Input: part model. Units: mm. Frame: model coordinates. Face numbers are marked on the shaded views. Coordinates: 2 decimals unless noted, no trailing zeros. Loops run counter-clockwise (first coordinate to the right, second up) from the corner with the lowest first, then second, coordinate; pieces in that order, holes last. Notation, with made-up numbers: M -5.75,16.25 L 26.25,16.25 A29 cw 26.25,42.25 Z; hole C -19,-20 d11. An arc over 180 degrees is marked long. Use a Markdown table: item, result. Add a question column.
1. Pin query (flat end, axial travel): pin 1 (7.5 mm diameter, centred on x = 7.5, z = 1.5, fed in from +Y). Return the tip coordinate at first contact, or that it passes through.
2. Section B-B on z = 0. Output: boundary loops of the cut face in (x, y), then the cut area to 3 significant figures.
3. Section A-A on y = 64.5. Output: boundary loops of the cut face in (x, z).
4. Section D-D on y = 47. Output: boundary loops of the cut face in (x, z).
5. Draft query along X for the marked faces 1, 2, 3 and 4. Return one class per face: +X half, -X half, draft (parallel to the pull), parting line (faces both ways), or undercut.
6. Section C-C on x = 17. Output: boundary loops of the cut face in (y, z).
7. Line query: L1, parallel to X at y = 7, z = 9.25; L2, parallel to Y at x = 3, z = 6.25; L3, parallel to Y at x = 20.6, z = 0. Output: solid intervals per line, ascending. Write a range as [from, to].
Autodesk Inventor part; units mm, degrees
ref_plane "YZ Plane" through (0, 0, 0) normal (1, 0, 0) x (0, 1, 0)
ref_plane "XZ Plane" through (0, 0, 0) normal (0, 1, 0) x (-1, 0, 0)
ref_plane "XY Plane" through (0, 0, 0) normal (0, 0, 1) x (1, 0, 0)
sketch "Sketch2" plane through (0, 0, 0) normal (0, 1, 0) x (-1, 0, 0)
  line L0 (-21.25, -13.75) -> (21.25, -13.75)
  line L1 (21.25, -13.75) -> (21.25, 13.75)
  line L2 (21.25, 13.75) -> (-21.25, 13.75)
  line L3 (-21.25, 13.75) -> (-21.25, -13.75)
  line L4 (-21.25, -13.75) -> (21.25, 13.75) construction
  line L5 (21.25, -13.75) -> (-21.25, 13.75) construction
  point P0 (0, 0)
  dimension "d2" = 42.5
  dimension "d3" = 27.5
extrude "Extrusion1" add sketch "Sketch2" against normal blind 2
sketch "Sketch3" plane through (0, 0, 0) normal (0, 1, 0) x (1, 0, 0)
  line L0 (21.25, -13.75) -> (-21.25, -13.75)
  line L1 (-21.25, 13.75) -> (21.25, 13.75)
  line L2 (-21.25, -13.75) -> (21.25, -13.75)
  line L3 (21.25, -13.75) -> (21.25, 13.75)
  line L4 (21.25, 13.75) -> (-21.25, 13.75)
  line L5 (-21.25, 13.75) -> (-21.25, -13.75)
  line L6 (-20.25, -12.75) -> (20.25, -12.75)
  line L7 (-20.25, 12.75) -> (-20.25, -12.75)
  line L8 (20.25, 12.75) -> (-20.25, 12.75)
  line L9 (20.25, -12.75) -> (20.25, 12.75)
  line L10 (-20.25, -12.75) -> (20.25, -12.75)
  line L11 (20.25, -12.75) -> (20.25, 12.75)
  line L12 (20.25, 12.75) -> (-20.25, 12.75)
  line L13 (-20.25, 12.75) -> (-20.25, -12.75)
  point P0 (0, 0)
extrude "Extrusion2" add sketch "Sketch3" along normal blind 60.5
fillet "Fillet1" radius 1 8 edges at (21.25, 29.25, 13.75) (21.25, 29.25, -13.75) (-21.25, 29.25, 13.75) (-21.25, 29.25, -13.75) (0, -2, -13.75) (21.25, -2, 0) (0, -2, 13.75) (-21.25, -2, 0)
sketch "Sketch4" plane through (0, 60.5, 0) normal (0, 1, 0) x (1, 0, 0)
  arc A0 (-20.25, 13.75) -> (-21.25, 12.75) centre (-20.25, 12.75) ccw
  line L0 (-21.25, 12.75) -> (-21.25, -12.75)
  arc A1 (-21.25, -12.75) -> (-20.25, -13.75) centre (-20.25, -12.75) ccw
  line L1 (-20.25, -13.75) -> (20.25, -13.75)
  arc A2 (20.25, -13.75) -> (21.25, -12.75) centre (20.25, -12.75) ccw
  line L2 (21.25, -12.75) -> (21.25, 12.75)
  arc A3 (21.25, 12.75) -> (20.25, 13.75) centre (20.25, 12.75) ccw
  line L3 (20.25, 13.75) -> (-20.25, 13.75)
  line L4 (-20.25, -12.75) -> (-20.25, 12.75)
  line L5 (-20.25, 12.75) -> (20.25, 12.75)
  line L6 (20.25, 12.75) -> (20.25, -12.75)
  line L7 (20.25, -12.75) -> (-20.25, -12.75)
  point P0 (0, 0)
extrude "Extrusion3" add sketch "Sketch4" along normal blind 8
sketch "Sketch5" plane through (21.25, -1, 12.75) normal (1, 0, 0) x (0, 0, -1)
  line L0 (26.5, 69.5) -> (25.5, 69.5)
  line L1 (-1, 69.5) -> (26.5, 69.5)
  line L2 (25.5, 69.5) -> (0, 69.5)
  line L3 (12.75, 69.5) -> (12.75, 61.5)
  circle A0 centre (12.75, 65.5) radius 1.25
  point P0 (12.75, 1)
  dimension "d11" = 8
  dimension "d12" = 2.5
extrude "Extrusion4" cut sketch "Sketch5" against normal through all
properties part number "Case"
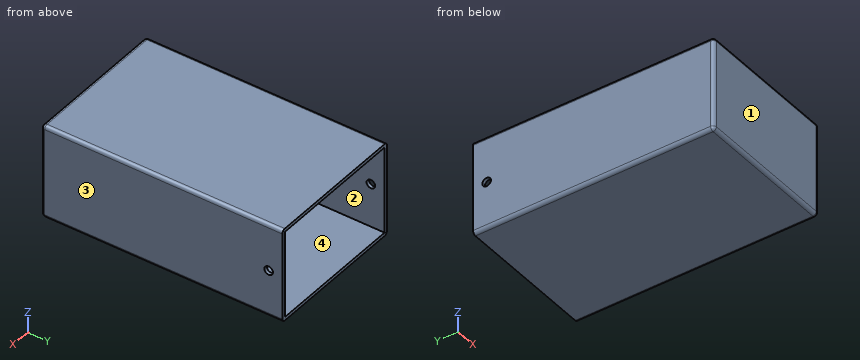
Answers below:
| question | item | result |
|---|---|---|
| 1 | pin 1 | stops at y = 0 |
| 2 | outline | M -21.25,-1 A1 ccw -20.25,-2 L 20.25,-2 A1 ccw 21.25,-1 L 21.25,63.25 L 20.25,63.25 L 20.25,0 L -20.25,0 L -20.25,63.25 L -21.25,63.25 Z; M -21.25,65.75 L -20.25,65.75 L -20.25,68.5 L -21.25,68.5 Z; M 20.25,65.75 L 21.25,65.75 L 21.25,68.5 L 20.25,68.5 Z |
| 2 | area | 217 mm² |
| 3 | outline | M -21.25,-12.75 A1 ccw -20.25,-13.75 L 20.25,-13.75 A1 ccw 21.25,-12.75 L 21.25,-1.25 L 20.25,-1.25 L 20.25,-12.75 L -20.25,-12.75 L -20.25,-1.25 L -21.25,-1.25 Z; M -21.25,1.25 L -20.25,1.25 L -20.25,12.75 L 20.25,12.75 L 20.25,1.25 L 21.25,1.25 L 21.25,12.75 A1 ccw 20.25,13.75 L -20.25,13.75 A1 ccw -21.25,12.75 Z |
| 4 | outline | M -21.25,-12.75 A1 ccw -20.25,-13.75 L 20.25,-13.75 A1 ccw 21.25,-12.75 L 21.25,12.75 A1 ccw 20.25,13.75 L -20.25,13.75 A1 ccw -21.25,12.75 Z; hole M -20.25,-12.75 L 20.25,-12.75 L 20.25,12.75 L -20.25,12.75 Z |
| 5 | face 1 | draft |
| 5 | face 2 | undercut |
| 5 | face 3 | +X half |
| 5 | face 4 | undercut |
| 6 | outline | M -2,-12.75 A1 ccw -1,-13.75 L 68.5,-13.75 L 68.5,-12.75 L 0,-12.75 L 0,12.75 L 68.5,12.75 L 68.5,13.75 L -1,13.75 A1 ccw -2,12.75 Z |
| 7 | L1 | x = [-21.25, -20.25], [20.25, 21.25] |
| 7 | L2 | y = [-2, 0] |
| 7 | L3 | y = [-1.94, 63.25], [65.75, 68.5] |
